```python
from build123d import *

# Parameters (mm, degrees)
SKETCH1_W                       = 51
SKETCH1_H                       = 39
SKETCH1_R                       = 1.75
SKETCH1_W_2                     = 33
SKETCH1_H_2                     = 23
BOSS_EXTRUDE1_DEPTH             = 4
FILLET1_R                       = 5
SKETCH2_W                       = 20.5
SKETCH2_H                       = 2
SKETCH2_W_2                     = 12
BOSS_EXTRUDE4_DEPTH             = 2
FILLET5_R                       = 5
CUT_EXTRUDE1_DEPTH              = 2.1
SKETCH5_W                       = 2
SKETCH5_H                       = 10
BOSS_EXTRUDE5_DEPTH             = 1
BOSS_EXTRUDE6_DEPTH             = 7
BOSS_EXTRUDE6_DEPTH_BACK        = 7
SKETCH7_R                       = 1.75
CUT_EXTRUDE2_DEPTH              = 5.394590795
BOSS_EXTRUDE7_REACH             = 61.994
SKETCH8_R                       = 1.75
SKETCH10_W                      = 11
SKETCH10_H                      = 4
BOSS_EXTRUDE9_DEPTH             = 20
BOSS_EXTRUDE9_DIRECTION_2_REACH = 91.634
SKETCH11_R                      = 1.75
CUT_EXTRUDE3_DEPTH              = 4


with BuildPart() as part:
    # Sketch1 → Boss-Extrude1 (new body)
    with BuildSketch(Plane(origin=(0, 0, 0), x_dir=(1, 0, 0), z_dir=(0, 1, 0))):
        with Locations((1, 0)):
            Rectangle(SKETCH1_W, SKETCH1_H)
        with Locations(Location((22.5, 7.25, 0), (0, 0, 270))):
            Circle(SKETCH1_R, mode=Mode.SUBTRACT)
        with Locations(Location((22.5, -7.25, 0), (0, 0, 90))):
            Circle(SKETCH1_R, mode=Mode.SUBTRACT)
        with Locations(Location((-14.5, -16, 0), (0, 0, 270))):
            Circle(SKETCH1_R, mode=Mode.SUBTRACT)
        Rectangle(SKETCH1_W_2, SKETCH1_H_2, mode=Mode.SUBTRACT)
    extrude(amount=BOSS_EXTRUDE1_DEPTH)

    # Fillet1
    fillet1_edges = [part.edges().sort_by_distance(p)[0] for p in [
        (-16.5, 2, -11.5),
        (-16.5, 2, 11.5),
        (16.5, 2, 11.5),
        (16.5, 2, -11.5),
    ]]
    fillet(fillet1_edges, radius=FILLET1_R)

    # Sketch2 → Boss-Extrude4 (add)
    with BuildSketch(Plane(origin=(0, 4, 0), x_dir=(1, 0, 0), z_dir=(0, 1, 0))):
        with Locations((-4.25, 13.8)):
            Rectangle(SKETCH2_W, SKETCH2_H)
        with Locations((0, -13.8)):
            Rectangle(SKETCH2_W_2, SKETCH2_H)
    extrude(amount=BOSS_EXTRUDE4_DEPTH)

    # Fillet5
    fillet5_edges = [part.edges().sort_by_distance(p)[0] for p in [
        (-24.5, 2, -19.5),
        (26.5, 2, -19.5),
        (26.5, 2, 19.5),
        (-24.5, 2, 19.5),
    ]]
    fillet(fillet5_edges, radius=FILLET5_R)

    # Sketch4 → Cut-Extrude1 (cut)
    with BuildSketch(Plane.XZ):
        Polygon((-12.854551733, 13.15), (-11.209103466, 16), (-12.854551733, 18.85), (-16.145448267, 18.85), (-17.790896534, 16), (-16.145448267, 13.15), align=None)
    extrude(amount=-CUT_EXTRUDE1_DEPTH, mode=Mode.SUBTRACT)

    # Sketch5 → Boss-Extrude5 (add)
    with BuildSketch(Plane(origin=(0, 4, 0), x_dir=(1, 0, 0), z_dir=(0, 1, 0))):
        with Locations((-19.1, 6.5)):
            Rectangle(SKETCH5_W, SKETCH5_H)
    extrude(amount=BOSS_EXTRUDE5_DEPTH)

    # Sketch6 → Boss-Extrude6 (add, two sides: drawn at the far end of the back side and taken through both)
    with BuildSketch(Plane.XY.offset(-BOSS_EXTRUDE6_DEPTH_BACK)):
        Polygon((-50.875844123, -25.455844123), (-25.42, 0), (-17.790896534, 0), (-47.06129239, -29.270395856), align=None)
    extrude(amount=BOSS_EXTRUDE6_DEPTH + BOSS_EXTRUDE6_DEPTH_BACK)

    # Sketch7 → Cut-Extrude2 (cut)
    with BuildSketch(Plane(origin=(-8.895448267, 8.895448267, 0), x_dir=(0, 0, -1), z_dir=(0.7071067811865489, -0.7071067811865462, 0))):
        with Locations(Location((0, -45.974654378, 0), (0, 0, 90))):
            Circle(SKETCH7_R)
    extrude(amount=-CUT_EXTRUDE2_DEPTH, mode=Mode.SUBTRACT)

    # Boss-Extrude7: up to this face of the body (flat: up to its plane)
    boss_extrude7_end = Plane(part.part.faces().sort_by_distance((-38.010311721, -12.590311721, 0))[0])
    # Sketch8 → Boss-Extrude7 (add, up to the picked face)
    with BuildSketch(Plane(origin=(-8.895448267, 8.895448267, 0), x_dir=(0, 0, -1), z_dir=(0.7071067811865489, -0.7071067811865462, 0)), mode=Mode.PRIVATE) as boss_extrude7_sk1:
        Polygon((7, -12.580063583), (33.15474804, -48.713282576), (25.054188906, -54.576808966), (7, -29.634647011), align=None)
        with Locations(Location((25, -45.974654378, 0), (0, 0, 90))):
            Circle(SKETCH8_R, mode=Mode.SUBTRACT)
    boss_extrude7_tool1 = split(extrude(boss_extrude7_sk1.sketch, amount=-BOSS_EXTRUDE7_REACH, mode=Mode.PRIVATE), bisect_by=boss_extrude7_end, keep=Keep.BOTH, mode=Mode.PRIVATE)
    add(boss_extrude7_tool1.solids().sort_by(Axis((-34.185622, -16.394725, -17.997204), (-0.7071067811865489, 0.7071067811865462, 0)))[0])

    # Sketch10 → Boss-Extrude9 (add)
    with BuildSketch(Plane(origin=(26.5, 0, 0), x_dir=(0, 0, -1), z_dir=(1, 0, 0))):
        with Locations((14, 2)):
            Rectangle(SKETCH10_W, SKETCH10_H)
    extrude(amount=BOSS_EXTRUDE9_DEPTH)

    # Sketch10 → Boss-Extrude9 direction 2 (add, up to next)
    with BuildSketch(Plane(origin=(26.5, 0, 0), x_dir=(0, 0, -1), z_dir=(1, 0, 0)), mode=Mode.PRIVATE) as boss_extrude9_direction_2_sk1:
        with Locations((14, 2)):
            Rectangle(SKETCH10_W, SKETCH10_H)
    boss_extrude9_direction_2_tool1 = extrude(boss_extrude9_direction_2_sk1.sketch, amount=-BOSS_EXTRUDE9_DIRECTION_2_REACH, mode=Mode.PRIVATE) - part.part
    add(boss_extrude9_direction_2_tool1.solids().sort_by_distance((26.5, 2, -14))[0])

    # Sketch11 → Cut-Extrude3 (cut)
    with BuildSketch(Plane(origin=(0, 4, 0), x_dir=(1, 0, 0), z_dir=(0, 1, 0))):
        with Locations(Location((38.97, 12, 0), (0, 0, 270))):
            Circle(SKETCH11_R)
    extrude(amount=-CUT_EXTRUDE3_DEPTH, mode=Mode.SUBTRACT)


solid = part.part
```
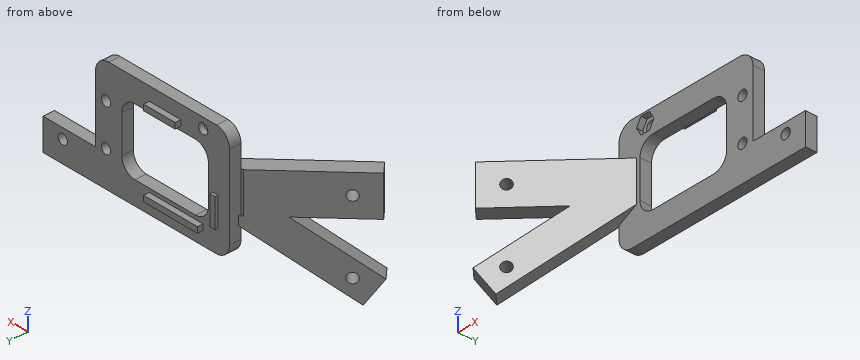
Here's how the part is built. I have some questions about the finished solid (model axes, mm). Give positions to 0.01 mm unless a question says otherwise; leave off trailing zeros. Order: outer loops, then holes, each group sorted by start corner. A loop starts at its lowest first (then second) coordinate and runs counter-clockwise, first axis right, second up. Notation, with made-up numbers: (63.25, 67) - (121.25, 67) arc R13 ccw to (121.25, 89) - close; hole circle Ø3 at (-29.5, 80.5). An arc over 180 degrees is marked (long way). Answer as a JSON object with one key per item and string values. Group by question number.
Item 1: If we section it at A-A on z = -4: Please give me the cut outline in (x, y), and give its area (3 significant figures).
Item 2: If we section it at B-B on x = -8: Please give me the cut outline in (y, z), and give its area (3 significant figures).
Item 3: For P1, Ø1.6, axis at y = 5, z = -13.5, coming from the -X side; P2, Ø12, axis at y = -23.5, z = -19.5, coming from the +X side; P3, Ø5.5, axis at x = -14.5, z = 16, coming from the +Y side, each with a flat end and sliding along its axis, tell me the tip position at first contact or that it passes through.
Item 4: Please list where these lines run through material, in increasing order: probe 1 along Y at (x, z) = (-8, -18); probe 2 along Z at (x, y) = (22, 3); probe 3 along Z at (x, y) = (38, 2).
Item 5: If we section it at C-C on y = -16: Please give me the cut outline in (x, z), and give its area (3 significant figures).
Item 6: If we section it at D-D on x = -35.5: Please give me the cut outline in (y, z), and give its area (3 significant figures).
Result set:
{
 "1": {"outline": "(-50.88, -25.46) - (-47.06, -29.27) - (-17.79, 0) - (-16.5, 0) - (-16.5, 4) - (-18.1, 4) - (-18.1, 5) - (-20.1, 5) - (-20.1, 4) - (-24.5, 4) - (-24.5, 0) - (-25.42, 0) - close; (16.5, 0) - (26.5, 0) - (26.5, 4) - (16.5, 4) - close", "area": "283 mm²"},
 "2": {"outline": "(0, -19.5) - (4, -19.5) - (4, -14.8) - (6, -14.8) - (6, -12.8) - (4, -12.8) - (4, -11.5) - (0, -11.5) - close; (0, 11.5) - (4, 11.5) - (4, 19.5) - (0, 19.5) - close", "area": "68.0 mm²"},
 "3": {"P1": "x = -14.5", "P2": "x = -35.29", "P3": "y = 4"},
 "4": {"probe 1": "0 to 4", "probe 2": "-19.5 to -8.93, -5.57 to 5.57, 8.93 to 19.47", "probe 3": "-19.5 to -13.46, -10.54 to -8.5"},
 "5": {"outline": "(-41.42, -27.28) - (-33.79, -23.38) - (-33.79, -11.03) - (-41.42, -14.94) - close; (-41.42, -7) - (-33.79, -7) - (-33.79, 7) - (-41.42, 7) - close", "area": "201 mm²"},
 "6": {"outline": "(-17.71, -25.13) - (-10.08, -21.22) - (-10.08, -8.88) - (-17.71, -12.78) - close; (-17.71, -7) - (-10.08, -7) - (-10.08, 7) - (-17.71, 7) - close", "area": "201 mm²"}
}
